Read the model definition and answer for the solid it produces. Units are mm, in the model's axes. Round coordinates to 2 decimals unless told otherwise and drop trailing zeros. Write each loop counter-clockwise with the first axis right and the second up, starting at its lowest first coordinate (ties: lowest second). Pieces come first, ordered by that corner, then holes. Notation, with made-up numbers: (71, -4) - (119, -4) arc R34 cw to (119, 34) - close; hole circle Ø4 at (-26, 55.25). An arc over 180 degrees is marked (long way). Answer as CSV lines item,"result". Start each with the question number.
1) Find section A-A on y = 0. Determine the outline of the cut face in (x, z) (1 decimal).
2) Find section B-B on x = -5.75. Determine the outline of the cut face in (y, z), then the cut area to 3 significant figures.
3) Find section D-D on x = 0. Determine the outline of the cut face in (y, z) (1 decimal), then the cut area to 3 significant figures.
4) Consider line 1 along Y through (x, z) = (0, 3.8) (3 decimals); line 2 along Y through (x, z) = (-4, 1.75); line 3 along X through (y, z) = (15.5, 3.55). Determine where each line is inside the solid, lowest interval first.
5) For a pull along X with two mould halves and no side action, classify faces 1 (the cylindrical face through (-9.2, -10.64, 2.35)), 2 (the cylindrical face through (9.3, -10.54, 2.35)), 3 (the flat face through (0, 13, 0)), 4 (the cylindrical face through (-0.2, 15.6, 3.7)) as +X half, -X half, draft (parallel to the pull), parting line (faces both ways), or undercut.
from build123d import *

# Parameters (mm, degrees)
SKETCH1_R                     = 9.525
BOSS_EXTRUDE2_DEPTH           = 4.7625
TAP_DRILL_FOR_6_32_TAP1_D     = 2.7051
TAP_DRILL_FOR_6_32_TAP1_DEPTH = 19.05
TAP_DRILL_FOR_6_32_TAP1_TIP   = 0.81269403


with BuildPart() as part:
    # Sketch1 → Boss-Extrude2 (new body)
    # profile 1 of 2: a face of its own
    with BuildSketch(Plane.XY):
        with BuildLine():
            Line((4.7625, 21.971), (-4.7625, 21.971))
            ThreePointArc((-4.7625, 21.971), (-9.252628061, 20.111128061), (-11.1125, 15.621))
            Line((-11.1125, 15.621), (-11.1125, 12.446))
            Line((-11.1125, 12.446), (11.1125, 12.446))
            Line((11.1125, 12.446), (11.1125, 15.621))
            ThreePointArc((11.1125, 15.621), (9.252628061, 20.111128061), (4.7625, 21.971))
        make_face()
    # profile 2 of 2: a face of its own
    with BuildSketch(Plane.XY):
        with BuildLine():
            Line((4.7625, -12.446), (-4.7625, -12.446))
            ThreePointArc((-4.7625, -12.446), (-9.252628061, -10.586128061), (-11.1125, -6.096))
            Line((-11.1125, -6.096), (-11.1125, 12.446))
            Line((-11.1125, 12.446), (11.1125, 12.446))
            Line((11.1125, 12.446), (11.1125, -6.096))
            ThreePointArc((11.1125, -6.096), (9.252628061, -10.586128061), (4.7625, -12.446))
        make_face()
        with Locations(Location((0, 0, 0), (0, 0, 180))):
            Circle(SKETCH1_R, mode=Mode.SUBTRACT)
    extrude(amount=BOSS_EXTRUDE2_DEPTH)

    # Tap Drill for #6-32 Tap1
    with Locations(Plane(origin=(0, 21.971, 0), x_dir=(1, 0, 0), z_dir=(0, 1, 0))):
        with Locations((-0.508, -2.38125)):
            Hole(TAP_DRILL_FOR_6_32_TAP1_D / 2, depth=TAP_DRILL_FOR_6_32_TAP1_DEPTH)
            with Locations((0, 0, -(TAP_DRILL_FOR_6_32_TAP1_DEPTH + TAP_DRILL_FOR_6_32_TAP1_TIP / 2))):  # 118° drill point
                Cone(0, TAP_DRILL_FOR_6_32_TAP1_D / 2, TAP_DRILL_FOR_6_32_TAP1_TIP, mode=Mode.SUBTRACT)


solid = part.part
Check values:
1,outline,"(-11.1, 0) - (-9.5, 0) - (-9.5, 4.8) - (-11.1, 4.8) - close; (9.5, 0) - (11.1, 0) - (11.1, 4.8) - (9.5, 4.8) - close"
2,outline,"(-12.37, 0) - (-7.59, 0) - (-7.59, 4.76) - (-12.37, 4.76) - close; (7.59, 0) - (21.89, 0) - (21.89, 4.76) - (7.59, 4.76) - close"
2,area,"90.8 mm^2"
3,outline,"(-12.4, 0) - (-9.5, 0) - (-9.5, 4.8) - (-12.4, 4.8) - close; (9.5, 0) - (22, 0) - (22, 1.1) - (9.5, 1.1) - close; (9.5, 3.6) - (22, 3.6) - (22, 4.8) - (9.5, 4.8) - close"
3,area,"42.0 mm^2"
4,line 1,"y = -12.446 to -9.525, 9.525 to 21.971"
4,line 2,"y = -12.45 to -8.64, 8.64 to 21.97"
4,line 3,"x = -11.11 to -1.19, 0.17 to 11.11"
5,face 1,"-X half"
5,face 2,"+X half"
5,face 3,"draft"
5,face 4,"undercut"
